Autodesk Inventor part; units mm, degrees
ref_plane "YZ Plane" through (0, 0, 0) normal (1, 0, 0) x (0, 1, 0)
ref_plane "XZ Plane" through (0, 0, 0) normal (0, 1, 0) x (-1, 0, 0)
ref_plane "XY Plane" through (0, 0, 0) normal (0, 0, 1) x (1, 0, 0)
sketch "スケッチ1" plane through (0, 0, 0) normal (0, 0, 1) x (1, 0, 0)
  circle A0 centre (0, 0) radius 8
  circle A1 centre (0, 0) radius 6
  circle A2 centre (0, 0) radius 1.25
  circle A3 centre (-2.8, -2.8) radius 1.5
  circle A4 centre (-2.8, 2.8) radius 1.5
  circle A5 centre (2.8, 2.8) radius 1.5
  circle A6 centre (2.8, -2.8) radius 1.5
  circle A7 centre (0, 0) radius 6
  dimension "d0" = 16
  dimension "d1" = 12
extrude "押し出し1" add sketch "スケッチ1" along normal blind 4.5 contours A1
properties part number "新型３脚最終段カム2" material "アルミニウム 2014-T4"
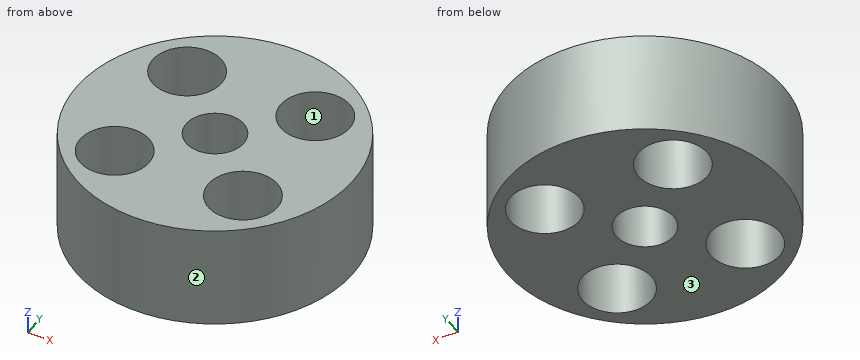
The model under review builds one solid part; all positions refer to its coordinate system, in mm. Face numbers are marked on the shaded views. Round coordinates to 2 decimals unless told otherwise and drop trailing zeros. Loops run counter-clockwise (first coordinate to the right, second up) from the corner with the lowest first, then second, coordinate; pieces in that order, holes last. Notation, with made-up numbers: (-15, 57) -> (21, 57) arc R21 ccw to (21, 75) -> close; hole circle Ø1 at (18.25, -26.5). An arc over 180 degrees is marked (long way). One line per question, with ' | ' between items. Start each with the question number.
Item 1: Add section B-B, the plane x = -2.5. Write out the cut boundary in (y, z).
Item 2: Add section C-C, the plane z = 2. Write out the cut boundary in (x, y), then the cut area to 3 significant figures.
Item 3: Wall thickness on line 1 along Y through (x, z) = (-2.8, 2.7); line 2 along Y through (x, z) = (-2, 4.2); line 3 along X through (y, z) = (0.75, 4.05): over which ranges is each line inside the solid? List them lowest first. Write a range as [from, to].
Item 4: Add section A-A, the plane y = 0. Write out the cut boundary in (x, z), then the cut area to 4 significant figures.
Item 5: Draft analysis for pull direction X (two halves, no side actions). For the marked faces 1, 2 and 3, state which applies: +X half, -X half, draft (parallel to the pull), parting line (faces both ways), or undercut.
Item 6: Add section D-D, the plane y = -1.5. Write out the cut boundary in (x, z), then the cut area to 3 significant figures.
Item 7: For pin 1 (2.5 mm diameter, centred on x = -2.8, y = -2.8, fed in from -Z); pin 2 (2 mm diameter, centred on y = 2.5, z = 1.5, fed in from -X); pin 3 (1.5 mm diameter, centred on y = -2, z = 2, fed in from -X), all flat-tipped, find the tip position at first contact; note any pin that passes through.
Return value:
1) outline: (-5.45, 0) -> (-4.27, 0) -> (-4.27, 4.5) -> (-5.45, 4.5) -> close; (-1.33, 0) -> (1.33, 0) -> (1.33, 4.5) -> (-1.33, 4.5) -> close; (4.27, 0) -> (5.45, 0) -> (5.45, 4.5) -> (4.27, 4.5) -> close
2) outline: circle Ø12 at (0, 0); hole circle Ø3 at (-2.8, -2.8); hole circle Ø3 at (-2.8, 2.8); hole circle Ø2.5 at (0, 0); hole circle Ø3 at (2.8, -2.8); hole circle Ø3 at (2.8, 2.8) | area: 79.9 mm2
3) line 1: y = [-5.31, -4.3], [-1.3, 1.3], [4.3, 5.31] | line 2: y = [-5.66, -4.07], [-1.53, 1.53], [4.07, 5.66] | line 3: x = [-5.95, -1], [1, 5.95]
4) outline: (-6, 0) -> (-1.25, 0) -> (-1.25, 4.5) -> (-6, 4.5) -> close; (1.25, 0) -> (6, 0) -> (6, 4.5) -> (1.25, 4.5) -> close | area: 42.75 mm2
5) face 1: undercut | face 2: parting line | face 3: draft
6) outline: (-5.81, 0) -> (-3.55, 0) -> (-3.55, 4.5) -> (-5.81, 4.5) -> close; (-2.05, 0) -> (2.05, 0) -> (2.05, 4.5) -> (-2.05, 4.5) -> close; (3.55, 0) -> (5.81, 0) -> (5.81, 4.5) -> (3.55, 4.5) -> close | area: 38.8 mm2
7) pin 1: passes through | pin 2: stops at x = -5.81 | pin 3: stops at x = -5.87
